```python
from build123d import *

# Parameters (mm, degrees)
CHAMFER1_SIZE = 0.5
CHAMFER2_SIZE = 0.2


with BuildPart() as part:
    # Sketch1 → Revolve1 (revolve)
    with BuildSketch(Plane(origin=(0, 0, 0), x_dir=(0, 0, -1), z_dir=(1, 0, 0))):
        with BuildLine():
            Line((77.5, 6), (77.5, 4))
            Line((77.5, 4), (119.5, 4))
            Line((119.5, 4), (119.5, 0))
            Line((119.5, 0), (-87.5, 0))
            Line((-87.5, 0), (-87.5, 4))
            Line((-87.5, 4), (-77.5, 4))
            Line((-77.5, 4), (-77.5, 5))
            Line((-77.5, 5), (-75, 5))
            Line((-75, 5), (-75, 14.7))
            ThreePointArc((-75, 14.7), (0, 15), (75, 14.7))
            Line((75, 14.7), (75, 6))
            Line((75, 6), (77.5, 6))
        make_face()
    revolve(axis=Axis((0, 0, -119.5), (0, 0, 1)))

    # Chamfer1
    chamfer1_edges = [part.edges().sort_by_distance(p)[0] for p in [
        (0, -4, 87.5),
        (0, -4, -119.5),
    ]]
    chamfer(chamfer1_edges, length=CHAMFER1_SIZE)

    # Chamfer2
    chamfer2_edges = [part.edges().sort_by_distance(p)[0] for p in [
        (0, -5, 77.5),
    ]]
    chamfer(chamfer2_edges, length=CHAMFER2_SIZE)


solid = part.part
```
Design review of the part built by this model. Coordinates are the model's own, in mm. A direction names the side the tool comes from. Round coordinates to 2 decimals unless told otherwise and drop trailing zeros. Write each loop counter-clockwise with the first axis right and the second up, starting at its lowest first coordinate (ties: lowest second). Pieces come first, ordered by that corner, then holes.
Item 1: Clearance check with flat-ended pins moving along their axes: pin 1 Ø3 at (x, y) = (-9, 7.5) entering from -Z; pin 2 Ø1 at (x, z) = (-11, -68) entering from -Y; pin 3 Ø4 at (x, z) = (2.5, -49.5) entering from +Y; pin 4 Ø10 at (y, z) = (11, -98) entering from -X. State where each tip first meets the part, or that it passes through.
Item 2: For faces 1 (the flat face through (6.3, -0.2, -75)), 2 (the flat face through (0, 0, -119.5)), 3 (the cylindrical face through (4.88, -1.08, 76.13)), list the 3-axis set-ups (+Z, -Z, +X, -X, +Y, -Y) from which the entire face can be reached by the end or side of a thin tool; tool diameter is ignored.
Item 3: For probe 1 along Z at (x, y) = (-1, 10.5); probe 2 along X at (y, z) = (-3, 19); probe 3 along Z at (x, y) = (-3.5, -4.5), list the stretches that pass through material, from the lowest coordinate up.
Item 4: We need section A-A on z = -88.5. Write out the cut boundary in (x, y).
Returned:
1. pin 1: stops at z = -75
1. pin 2: stops at y = -10.36
1. pin 3: stops at y = 14.86
1. pin 4: passes through
2. face 1: -Z
2. face 2: -Z, +X, -X, +Y, -Y
2. face 3: +Z
3. probe 1: z = -75 to 75
3. probe 2: x = -14.68 to 14.68
3. probe 3: z = -77.5 to 75
4. outline: circle Ø8 at (0, 0)
